Print and shaded views of the part. All mm, measured from the part's lowest x, y and z. Give positions to 0.01 mm unless a question says otherwise; leave off trailing zeros. Loops run counter-clockwise (first coordinate to the right, second up) from the corner with the lowest first, then second, coordinate; pieces in that order, holes last. Notation, with made-up numbers: (69.5, -16.75) -> (123.5, -16.75) arc R19 cw to (123.5, -5.75) -> close; hole circle Ø2 at (17.5, -13). An arc over 180 degrees is marked (long way). Answer as a JSON object with one key per item and string values. Group by question number.
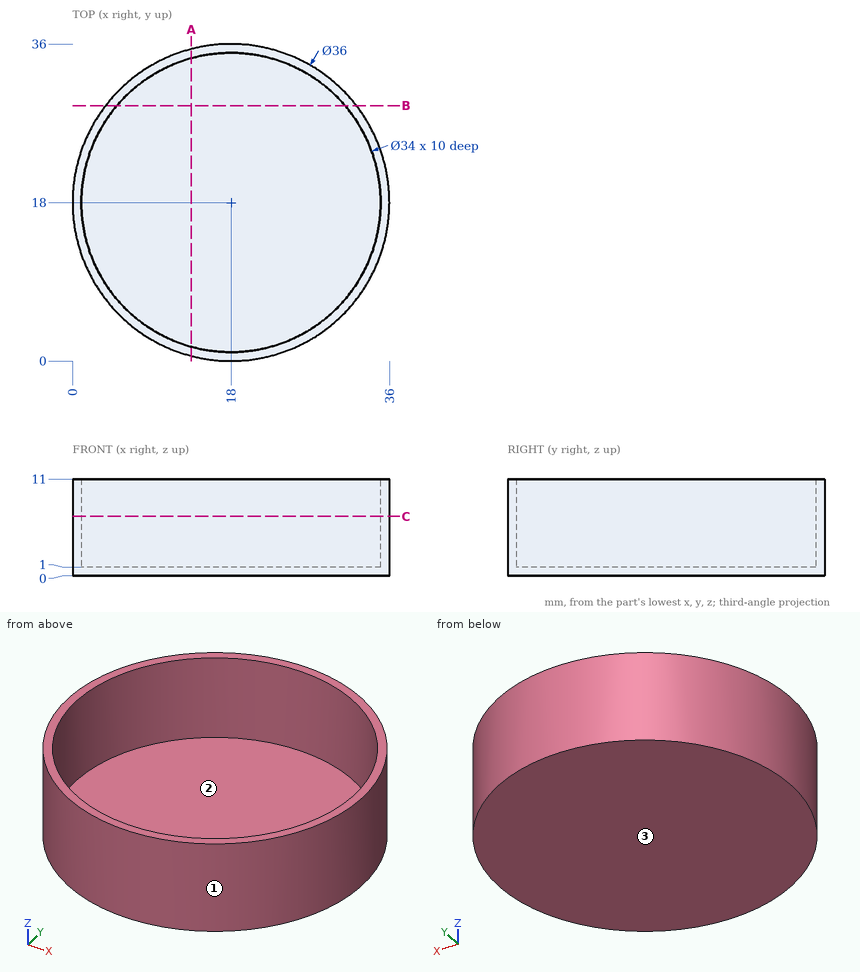
(1) Saw through at C-C on z = 6.75. List the corners of the cut face in (x, y), plus the area to 3 significant figures.
(2) Saw through at A-A on x = 13.5. List the corners of the cut face in (y, z), plus the area to 3 significant figures.
(3) Pin check, flat tips, straight feed: pin 1 (1 mm diameter, centred on x = 8.5, y = 12, fed in from +Z); pin 2 (6 mm diameter, centred on y = 6.5, z = 8.5, fed in from -X); pin 3 (6 mm diameter, centred on y = 4, z = 2, fed in from -X). Stop position of each tip, or through.
(4) Probe line 1 along Y through (x, z) = (18, 5); line 2 along Z through (x, y) = (22.5, 33); line 3 along X through (y, z) = (10, 5.25). List the from-to ranges inside material, lowest first. Write a range as [from, to].
(5) Pull direction X, two halves, no side cores. Call the marked faces 1, 2 and 3: pulls with the +X half, pulls with the -X half, needs draft (parallel to the pull), parting line crosses it, or undercut.
(6) Saw through at B-B on y = 29. List the corners of the cut face in (x, z), plus the area to 3 significant figures.
Calculated:
{
 "1": {"outline": "circle Ø36 at (18, 18); hole circle Ø34 at (18, 18)", "area": "110 mm^2"},
 "2": {"outline": "(0.57, 0) -> (35.43, 0) -> (35.43, 11) -> (34.39, 11) -> (34.39, 1) -> (1.61, 1) -> (1.61, 11) -> (0.57, 11) -> close", "area": "55.6 mm^2"},
 "3": {"pin 1": "stops at z = 1", "pin 2": "stops at x = 2.13", "pin 3": "stops at x = 3.75"},
 "4": {"line 1": "y = [0, 1], [35, 36]", "line 2": "z = [0, 1]", "line 3": "x = [1.88, 3], [33, 34.12]"},
 "5": {"face 1": "parting line crosses it", "face 2": "undercut", "face 3": "needs draft"},
 "6": {"outline": "(3.75, 0) -> (32.25, 0) -> (32.25, 11) -> (30.96, 11) -> (30.96, 1) -> (5.04, 1) -> (5.04, 11) -> (3.75, 11) -> close", "area": "54.2 mm^2"}
}
